Could you check a few things on this model? Use its own coordinates, in mm. A direction names the side the tool comes from. Coordinates: 2 decimals unless noted, no trailing zeros. Order: outer loops, then holes, each group sorted by start corner. A loop starts at its lowest first (then second) coordinate and runs counter-clockwise, first axis right, second up. Notation, with made-up numbers: (72.25, 80) -> (123.25, 80) arc R14 ccw to (123.25, 104) -> close; hole circle Ø4 at (-37.5, 4.5). An arc over 180 degrees is marked (long way). Use a Markdown table: item, result. Add a question column.
1) If we section it at A-A (z = -6.5): Write out the boundary of the cut face in (x, y), plus the area to 3 significant figures.
2) Which directions (+Z, -Z, +X, -X, +Y, -Y) give clear straight access to the entire face, cutting with the end or side of a thin tool? Please do faces 4 (the flat face through (-224, -1, -9)), 5 (the flat face through (-53, 1, 0)), 6 (the flat face through (3, -84, -25)), 7 (the cylindrical face through (224.493, -49.997, -24.725)).
3) Thinking about a two-plate mould opening in X: for faces 1 (the flat face through (224, -1, -9)), 2 (the flat face through (-53, 1, 1)), 3 (the flat face through (-225, -1, -41)), which applies, +X half, -X half, draft (parallel to the pull), parting line (faces both ways), or undercut?
4) If we section it at D-D (z = -25): Write out the boundary of the cut face in (x, y).
5) Will these pins go through, and if not, where does the flat tip stop? pin 1 Ø1 at (x, z) = (224.5, -20.5) entering from +Y; pin 2 Ø1 at (x, z) = (224, -15.5) entering from -Y; pin 3 Ø0.6 at (y, z) = (84.5, -35.5) entering from -X.
6) If we section it at C-C (y = 0): Give the number of separate pieces and of enclosed holes in the cut face, plus the area to 3 significant figures.
7) If I drill on L1, parallel to X at y = -9.5, z = -42.5; L2, parallel to Y at x = -140, z = -30; L3, parallel to Z at x = -27, y = -73, over which ranges is the centre line in solid material (lowest first)? Write a range as [from, to].
8) If we section it at B-B (x = 150): Write out the boundary of the cut face in (y, z).
```python
from build123d import *

# Parameters (mm, degrees)
F3_W           = 446
F3_H           = 166
F3_R           = 50
F4_DEPTH       = 1
F6_DEPTH       = 223
F8_DEPTH       = 83
F10_DEPTH      = 225.001
F10_DEPTH_BACK = 225.001


# Not quite as in the source:
# - a pattern or mirror of a feature is missing from the dataset's text; its kind, count and spacing are read off the source's solid


with BuildPart() as f4:
    # F3 (on Top) → F4 (new body)
    with BuildSketch(Plane.XY):
        Rectangle(F3_W, F3_H)
        with Locations((-150, 0)):
            Circle(F3_R, mode=Mode.SUBTRACT)
        Circle(F3_R, mode=Mode.SUBTRACT)
        with Locations((150, 0)):
            Circle(F3_R, mode=Mode.SUBTRACT)
    extrude(amount=F4_DEPTH)

    # F5 (on Right) → F6 (join, symmetric)
    with BuildSketch(Plane.YZ):
        with BuildLine():
            ThreePointArc((85, -1), (84.4142135624, 0.4142135624), (83, 1))
            Line((83, 1), (83, 0))
            ThreePointArc((83, 0), (83.7071067812, -0.2928932188), (84, -1))
            Line((84, -1), (84, -49))
            Line((84, -49), (85, -49))
            Line((85, -49), (85, -1))
        make_face()
    f6 = extrude(amount=F6_DEPTH, both=True)

    # F6_copies: F6 across plane
    add(f6.mirror(Plane(origin=(0, 0, 0), x_dir=(0, 0, -1), z_dir=(0, -1, 0))))

    # F7 (on Front) → F8 (join, symmetric)
    with BuildSketch(Plane.XZ):
        with BuildLine():
            ThreePointArc((225, -1), (224.4142135624, 0.4142135624), (223, 1))
            Line((223, 1), (223, 0))
            ThreePointArc((223, 0), (223.7071067812, -0.2928932188), (224, -1))
            Line((224, -1), (224, -49))
            Line((224, -49), (225, -49))
            Line((225, -49), (225, -1))
        make_face()
    f8 = extrude(amount=F8_DEPTH, both=True)

    # F8_copies: F8 across plane
    add(f8.mirror(Plane(origin=(0, 0, 0), x_dir=(0, 0, -1), z_dir=(-1, 0, 0))))

    # F9 (on Right) → F10 (cut, two sides)
    with BuildSketch(Plane.YZ) as f10_sk:
        with BuildLine():
            ThreePointArc((37.5, -37.5), (50, -25), (37.5, -12.5))
            Line((37.5, -12.5), (-37.5, -12.5))
            ThreePointArc((-37.5, -12.5), (-50, -25), (-37.5, -37.5))
            Line((-37.5, -37.5), (37.5, -37.5))
        make_face()
    extrude(amount=-F10_DEPTH, mode=Mode.SUBTRACT)
    extrude(f10_sk.sketch, amount=F10_DEPTH_BACK, mode=Mode.SUBTRACT)


solid = f4.part
```
Answer sheet:
| question | item | result |
|---|---|---|
| 1 | outline | (-225, -83) -> (-224, -83) -> (-224, 83) -> (-225, 83) -> close; (-223, -85) -> (223, -85) -> (223, -84) -> (-223, -84) -> close; (-223, 84) -> (223, 84) -> (223, 85) -> (-223, 85) -> close; (224, -83) -> (225, -83) -> (225, 83) -> (224, 83) -> close |
| 1 | area | 1,220 mm2 |
| 2 | face 4 | -Z, +Y, -Y |
| 2 | face 5 | -Z |
| 2 | face 6 | -Z, +X, -X |
| 2 | face 7 | +X, -X |
| 3 | face 1 | undercut |
| 3 | face 2 | draft |
| 3 | face 3 | -X half |
| 4 | outline | (-225, -83) -> (-224, -83) -> (-224, -50) -> (-225, -50) -> close; (-225, 50) -> (-224, 50) -> (-224, 83) -> (-225, 83) -> close; (-223, -85) -> (223, -85) -> (223, -84) -> (-223, -84) -> close; (-223, 84) -> (223, 84) -> (223, 85) -> (-223, 85) -> close; (224, -83) -> (225, -83) -> (225, -50) -> (224, -50) -> close; (224, 50) -> (225, 50) -> (225, 83) -> (224, 83) -> close |
| 5 | pin 1 | y = 83 |
| 5 | pin 2 | y = -83 |
| 5 | pin 3 | x = -223 |
| 6 | separate pieces | 6 |
| 6 | enclosed holes | 0 |
| 6 | area | 197 mm2 |
| 7 | L1 | [-225, -224], [224, 225] |
| 7 | L2 | [-85, -84], [84, 85] |
| 7 | L3 | [0, 1] |
| 8 | outline | (-85, -49) -> (-84, -49) -> (-84, -1) arc R1 cw to (-83, 0) -> (-50, 0) -> (-50, 1) -> (-83, 1) arc R2 ccw to (-85, -1) -> close; (50, 0) -> (83, 0) arc R1 cw to (84, -1) -> (84, -49) -> (85, -49) -> (85, -1) arc R2 ccw to (83, 1) -> (50, 1) -> close |
